Model file for the job. Use its own axes, mm. Give positions to 0.01 mm unless a question says otherwise; leave off trailing zeros. Order: outer loops, then holes, each group sorted by start corner. A loop starts at its lowest first (then second) coordinate and runs counter-clockwise, first axis right, second up. Notation, with made-up numbers: (61, 14) - (68, 14) arc R9 ccw to (68, 30) - close; hole circle Ø6 at (70.25, 25). An arc over 180 degrees is marked (long way). Return JSON: item names as keys, results as strings. Group by question number.
from build123d import *

# Parameters (mm, degrees)
SKETCH1_R           = 7.9375
BOSS_EXTRUDE1_DEPTH = 127
CUT_EXTRUDE1_DEPTH  = 128


with BuildPart() as part:
    # Sketch1 → Boss-Extrude1 (new body)
    with BuildSketch(Plane.XY):
        Circle(SKETCH1_R)
    extrude(amount=BOSS_EXTRUDE1_DEPTH)

    # Sketch2 → Cut-Extrude1 (cut, through all)
    with BuildSketch(Plane.XY.offset(127)):
        Polygon((0, 1.5875), (1.5875, 1.5875), (1.5875, -1.5875), (-1.5875, -1.5875), (-1.5875, 1.5875), align=None)
    extrude(amount=-CUT_EXTRUDE1_DEPTH, mode=Mode.SUBTRACT)


solid = part.part
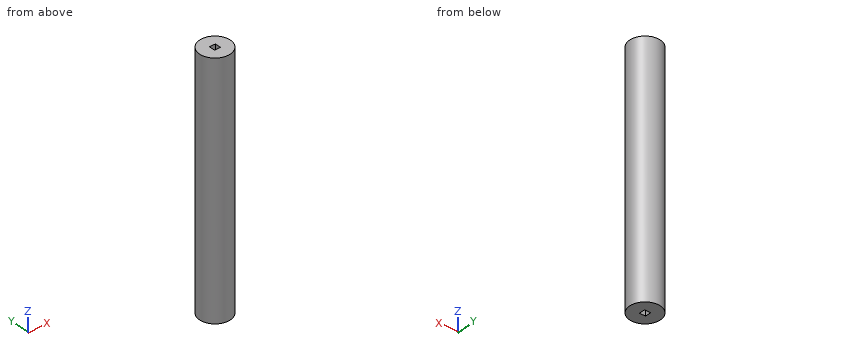
(1) Slice it at D-D (y = -6.5). Give the cut face in (x, z).
(2) Slice it at C-C (z = 34.5). Give the cut face in (x, y) (1 decimal).
(3) Slice it at A-A (x = 0). Give the cut face in (y, z).
(4) Drill centre lines: L1, parallel to Y at x = -1, z = 26; L2, parallel to X at y = 7, z = 115; L3, parallel to Y at x = 2.5, z = 34.5. Where is each one in solid material? Low to high.
(5) Drop flat-ended pins along their axis: pin 1 Ø1 at (x, z) = (5, 49) entering from +Y; pin 2 Ø1 at (x, z) = (3, 41) entering from -Y; pin 3 Ø1.5 at (y, z) = (4, 32) entering from +X. Give the stop position or say it passes through.
Result set:
{
 "1": {"outline": "(-4.56, 0) - (4.56, 0) - (4.56, 127) - (-4.56, 127) - close"},
 "2": {"outline": "circle Ø15.9 at (0, 0); hole (-1.6, -1.6) - (1.6, -1.6) - (1.6, 1.6) - (-1.6, 1.6) - close"},
 "3": {"outline": "(-7.94, 0) - (-1.59, 0) - (-1.59, 127) - (-7.94, 127) - close; (1.59, 0) - (7.94, 0) - (7.94, 127) - (1.59, 127) - close"},
 "4": {"L1": "y = -7.87 to -1.59, 1.59 to 7.87", "L2": "x = -3.74 to 3.74", "L3": "y = -7.53 to 7.53"},
 "5": {"pin 1": "stops at y = 6.54", "pin 2": "stops at y = -7.53", "pin 3": "stops at x = 7.24"}
}
